from build123d import *

# Parameters (mm, degrees)
EXTRUDE_376_DEPTH   = 10
SKETCH_2_OUTSIDE_W  = 172.148
SKETCH_2_OUTSIDE_H  = 175.86
SKETCH_2_OUTSIDE_R  = 11.994451842
CUT_EXTRUDE_1_DEPTH = 40
CUT_EXTRUDE_1_DRAFT = -60
SKETCH_3_R          = 8
EXTRUDE_1_DEPTH     = 50
CHAMFER_1_SIZE      = 1.5
FILLET_1_R          = 1


with BuildPart() as part:
    # Эскиз1 → Extrude 376 (new body)
    with BuildSketch(Plane.XY):
        Polygon((-11.994451842, 6.925), (0, 13.85), (11.994451842, 6.925), (11.994451842, -6.925), (0, -13.85), (-11.994451842, -6.925), align=None)
    extrude(amount=EXTRUDE_376_DEPTH)


with BuildPart() as cut_extrude_1_tool:
    # Эскиз2 outside → Вырез-Вытянуть1 (with draft: the straight prism first)
    with BuildSketch(Plane.XY.offset(10)):
        Rectangle(SKETCH_2_OUTSIDE_W, SKETCH_2_OUTSIDE_H)
        Circle(SKETCH_2_OUTSIDE_R, mode=Mode.SUBTRACT)
    extrude(amount=-CUT_EXTRUDE_1_DEPTH)
    # Вырез-Вытянуть1: the draft: its side faces are tilted about the plane it starts from
    cut_extrude_1_sides = [cut_extrude_1_tool.faces().sort_by_distance(p)[0] for p in [
        (0, -87.93, -10),
        (86.074, 0, -10),
        (0, 87.93, -10),
        (-86.074, 0, -10),
        (-11.994451842, 0, -10),
    ]]
    draft(cut_extrude_1_sides, Plane.XY.offset(10), CUT_EXTRUDE_1_DRAFT)


with BuildPart() as part_1:
    add(part.part)

    # Вырез-Вытянуть1: cut by cut_extrude_1_tool
    add(cut_extrude_1_tool.part, mode=Mode.SUBTRACT)

    # Эскиз3 → Бобышка-Вытянуть1 (add)
    with BuildSketch(Plane(origin=(0, 0, 0), x_dir=(-1, 0, 0), z_dir=(0, 0, -1))):
        Circle(SKETCH_3_R)
    extrude(amount=EXTRUDE_1_DEPTH)

    # Фаска1
    chamfer_1_edges = [part_1.edges().sort_by_distance(p)[0] for p in [
        (8, 0, -50),
    ]]
    chamfer(chamfer_1_edges, length=CHAMFER_1_SIZE)

    # Скругление1
    fillet_1_edges = [part_1.edges().sort_by_distance(p)[0] for p in [
        (8, 0, 0),
    ]]
    fillet(fillet_1_edges, radius=FILLET_1_R)


solid = part_1.part
Build history of the part. All positions in model axes, mm. A direction names the side the tool comes from. Give positions to 0.01 mm unless a question says otherwise; leave off trailing zeros. Order: outer loops, then holes, each group sorted by start corner. A loop starts at its lowest first (then second) coordinate and runs counter-clockwise, first axis right, second up. Notation, with made-up numbers: M 38.5,88 L 45.5,88 A25 ccw 45.5,108 Z; hole C 6.5,-26 d7. An arc over 180 degrees is marked long. Put each result on its own line as item: value.
Item 1: 3-axis set-ups, long thin cutter, end or side, ignore diameter. For faces 1 (the conical face through (-10.786, -6.192, 9.745)), 2 (the cylindrical face through (1.73, -7.81, -24.42)): which of +Z, -Z, +X, -X, +Y, -Y reach the whole face in a straight line?
From the geometry:
face 1: +Z, -X, -Y
face 2: -Z
Item 2: Flat gauge pins, fed straight in: pin 1 Ø1 at (y, z) = (-4, -29) entering from -X; pin 2 Ø1 at (x, z) = (-6, -2) entering from -Y; pin 3 Ø12 at (x, z) = (-3.5, -12) entering from -Y; pin 4 Ø1.5 at (x, z) = (9, -35) entering from +Y. Where does each tip first touch, or does it go through?
From the geometry:
pin 1: stops at x = -7.19
pin 2: stops at y = -5.81
pin 3: stops at y = -8
pin 4: passes through
Item 3: Slice it at A-A, the plane z = -4. Write the cut outline in (x, y), plus the area to 3 significant figures.
From the geometry:
outline: C 0,0 d16
area: 201 mm2
Item 4: Probe line 1 (Z direction, x = 3.25, y = 8.25); line 2 (Y direction, x = -4, z = -34); line 3 (X direction, y = -3.5, z = -26). List the from-to ranges inside material, lowest first. Write a range as [from, to].
From the geometry:
line 1: z = [-0.01, 10]
line 2: y = [-6.93, 6.93]
line 3: x = [-7.19, 7.19]
